```python
from build123d import *

# Parameters (mm, degrees)
SKETCH3_R               = 10.16
BOSS_EXTRUDE2_DEPTH     = 12.7
BOSS_EXTRUDE3_DEPTH     = 50.8
CUT_EXTRUDE1_DEPTH      = 195.200593167
CUT_EXTRUDE1_DEPTH_BACK = 195.200593167


with BuildPart() as part:
    # Sketch3 → Boss-Extrude2 (new body)
    # profile 1 of 2: a face of its own
    with BuildSketch(Plane(origin=(0, 0, 0), x_dir=(1, 0, 0), z_dir=(0, 1, 0))):
        with BuildLine():
            Line((0, 57.15), (0, 35.56))
            Line((0, 35.56), (25.4, 35.56))
            ThreePointArc((25.4, 35.56), (35.56, 25.4), (25.4, 15.24))
            Line((25.4, 15.24), (0, 15.24))
            Line((0, 15.24), (0, 0))
            Line((0, 0), (152.4, 0))
            Line((152.4, 0), (152.4, 57.15))
            Line((152.4, 57.15), (0, 57.15))
        make_face()
        with Locations(Location((127, 25.4, 0), (0, 0, 270))):
            Circle(SKETCH3_R, mode=Mode.SUBTRACT)
    # profile 2 of 2: a face of its own
    with BuildSketch(Plane(origin=(0, 0, 0), x_dir=(1, 0, 0), z_dir=(0, 1, 0))):
        with BuildLine():
            Line((0, 78.74), (0, 57.15))
            Line((0, 57.15), (152.4, 57.15))
            Line((152.4, 57.15), (152.4, 114.3))
            Line((152.4, 114.3), (0, 114.3))
            Line((0, 114.3), (0, 99.06))
            Line((0, 99.06), (25.4, 99.06))
            ThreePointArc((25.4, 99.06), (35.56, 88.9), (25.4, 78.74))
            Line((25.4, 78.74), (0, 78.74))
        make_face()
        with Locations(Location((127, 88.9, 0), (0, 0, 270))):
            Circle(SKETCH3_R, mode=Mode.SUBTRACT)
    extrude(amount=-BOSS_EXTRUDE2_DEPTH)

    # Sketch4 → Boss-Extrude3 (add)
    with BuildSketch(Plane(origin=(0, 0, 0), x_dir=(1, 0, 0), z_dir=(0, 1, 0))):
        Polygon((76.2, 0), (19.05, 50.401562476), (69.451562476, 107.551562476), (126.601562476, 57.15), align=None)
    extrude(amount=BOSS_EXTRUDE3_DEPTH)

    # Sketch5 → Cut-Extrude1 (cut, two sides: drawn at the far end of the back side and taken through both)
    with BuildSketch(Plane(origin=(42.8625, 0, 37.801171857), x_dir=(0.661437827766148, 0, -0.7499999999999998), z_dir=(0.7499999999999998, 0, 0.661437827766148)).offset(-CUT_EXTRUDE1_DEPTH_BACK)):
        Polygon((56.751562476, 50.8), (85.326562476, 22.225), (85.326562476, 15.875), (91.676562476, 15.875), (91.676562476, 22.225), (120.251562476, 50.8), align=None)
    extrude(amount=CUT_EXTRUDE1_DEPTH + CUT_EXTRUDE1_DEPTH_BACK, mode=Mode.SUBTRACT)


solid = part.part
```
Geometry check sheet. Reference: the model listing, model coordinates, mm. A direction names the side the tool comes from. Round coordinates to 2 decimals unless told otherwise and drop trailing zeros. Loops run counter-clockwise (first coordinate to the right, second up) from the corner with the lowest first, then second, coordinate; pieces in that order, holes last. Notation, with made-up numbers: (-4.5, 56) - (26.5, 56) arc R17 ccw to (26.5, 62) - close; hole circle Ø4 at (7.25, 25). An arc over 180 degrees is marked (long way). Write each question's results on one line, items separated by ' | '. Start each with the question number.
Q1. Cross-section at A-A on z = -24. Enter the section's corners in (x, y), and give its area (3 significant figures).
Q2. Access from +Z, -Z, +X, -X, +Y, -Y to the whole of each face (thin tool, end or side, straight path). Record for faces 1 (the flat face through (48.025, 25.044, -24.848)), 2 (the flat face through (70.326, 19.094, -51.747)), 3 (the flat face through (13, -6, -15.24)).
Q3. Cross-section at B-B on y = 42.5. Enter the section's corners in (x, z), and give its area (3 significant figures).
Q4. Gauge pin test, flat ends, axial feed: P1, Ø1, axis at y = 20, z = -83, coming from the +X side; P2, Ø4, axis at y = 24.5, z = -86, coming from the +X side; P3, Ø6, axis at y = 18, z = -63, coming from the -X side (3 decimals). Record the tip position at first contact, or that the pin passes through.
Q5. Thickness scan on line 1 (X direction, y = -9, z = -25); line 2 (Y direction, x = 129, z = -75.5); line 3 (Z direction, x = 52.5, y = 17). Record the ranges inside material, lowest first. Write a range as [from, to].
Q6. Cross-section at D-D on x = 72.5. Enter the section's corners in (y, z) (3 decimals), and give its area (3 significant figures).
Q7. Release check for a two-part mould opening along Z. For faces 4 (the flat face through (13, -6, -99.06)), 5 (the flat face through (101.754, 13.756, -28.975)), 6 (the flat face through (98, 50.8, -78)), 7 (the flat face through (97.63, 25.04, -82.7)) record: +Z half, -Z half, draft (parallel to the pull), parting line (faces both ways), or undercut.
Q8. Cross-section at C-C on y = -6. Enter the section's corners in (x, z), and give its area (3 significant figures).
Answers below:
1) outline: (35.46, -12.7) - (116.94, -12.7) - (116.94, 0) - (97.37, 0) - (97.37, 25.15) - (58.59, 50.8) - (48.99, 50.8) - (48.99, 0) - (35.46, 0) - close; (137.06, -12.7) - (152.4, -12.7) - (152.4, 0) - (137.06, 0) - close | area: 3,190 mm²
2) face 1: +Z, -X, +Y | face 2: +Y | face 3: -X, +Y, -Y
3) outline: (19.05, -50.4) - (28.74, -61.39) - (85.89, -10.99) - (76.2, 0) - close; (59.76, -96.56) - (69.45, -107.55) - (126.6, -57.15) - (116.91, -46.16) - close | area: 2,230 mm²
4) P1: stops at x = 97.86 | P2: stops at x = 96.16 | P3: stops at x = 27.515
5) line 1: x = [35.55, 116.85], [137.15, 152.4] | line 2: y = [-12.7, 0] | line 3: z = [-88.33, -75.93], [-67.47, -20.9]
6) outline: (-12.7, -114.3) - (0, -114.3) - (0, -104.863) - (50.8, -104.863) - (50.8, -96.396) - (22.225, -58.296) - (15.875, -58.296) - (15.875, -49.83) - (22.225, -49.83) - (50.8, -11.73) - (50.8, -3.263) - (0, -3.263) - (0, 0) - (-12.7, 0) - close | area: 5,230 mm²
7) face 4: undercut | face 5: +Z half | face 6: draft | face 7: -Z half
8) outline: (0, -114.3) - (152.4, -114.3) - (152.4, 0) - (0, 0) - (0, -15.24) - (25.4, -15.24) arc R10.16 cw to (25.4, -35.56) - (0, -35.56) - (0, -78.74) - (25.4, -78.74) arc R10.16 cw to (25.4, -99.06) - (0, -99.06) - close; hole circle Ø20.32 at (127, -88.9); hole circle Ø20.32 at (127, -25.4) | area: 15,400 mm²
